Could you check a few things on this drawing? It's one solid part, dimensions in mm from its lowest x, y, z. A direction names the side the tool comes from. Round coordinates to 2 decimals unless told otherwise and drop trailing zeros. Write each loop counter-clockwise with the first axis right and the second up, starting at its lowest first coordinate (ties: lowest second). Pieces come first, ordered by that corner, then holes. Notation, with made-up numbers: M 75,2 L 86,2 A22 cw 86,18 Z; hole C 72.5,46 d5. An arc over 180 degrees is marked long. One line per item, written item: value. Start each with the question number.
(1) I want a section at D-D on y = 23. Please give me the cut outline in (x, z).
(2) If I drill on L1, parallel to X at y = 6, z = 135; L2, parallel to X at y = 1.45, z = 103; L3, parallel to Z at x = 10, y = 11.5, over which ranges is the centre line in solid material (lowest first)?
(3) I'm going to push flat-ended pins straight in: pin 1 Ø5 at (x, z) = (15.5, 42) entering from +Y; pin 2 Ø2.5 at (x, z) = (16, 103) entering from -Y; pin 3 Ø1 at (x, z) = (21.5, 145) entering from +Y. Where does each tip first touch, or does it pass through?
(4) I want a section at C-C on z = 103. Please give me the cut outline in (x, y).
(5) I want a section at B-B on y = 8. Please give me the cut outline in (x, z), and give its area (3 significant figures).
(6) Which directions (+Z, -Z, +X, -X, +Y, -Y) give clear straight access to the entire face, cutting with the end or side of a thin tool? Please do the marked faces 1 and 2.
(7) Thinking about a two-plate mould opening in X: for the marked faces 3, 4 and 5, which applies, released by +X, released by -X, zero draft, split by the parting line, or undercut?
(8) I want a section at A-A on x = 16. Please give me the cut outline in (y, z).
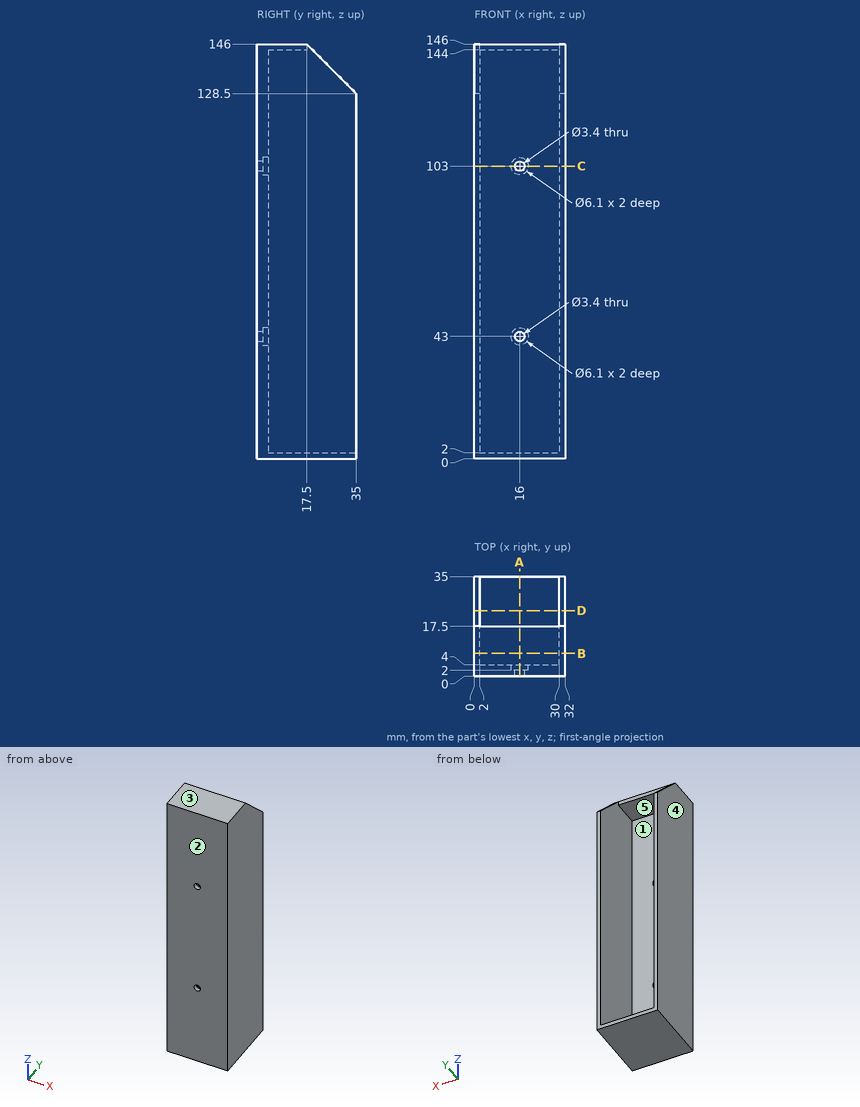
Found:
1. outline: M 0,0 L 32,0 L 32,140.5 L 30,140.5 L 30,2 L 2,2 L 2,140.5 L 0,140.5 Z
2. L1: x = 0 to 2, 30 to 32
2. L2: x = 0 to 14.3, 17.7 to 32
2. L3: z = 0 to 2, 144 to 146
3. pin 1: stops at y = 4
3. pin 2: passes through
3. pin 3: stops at y = 17.5
4. outline: M 0,0 L 14.3,0 L 14.3,2 L 12.95,2 L 12.95,4 L 2,4 L 2,35 L 0,35 Z; M 17.7,0 L 32,0 L 32,35 L 30,35 L 30,4 L 19.05,4 L 19.05,2 L 17.7,2 Z
5. outline: M 0,0 L 32,0 L 32,146 L 0,146 Z; hole M 2,2 L 30,2 L 30,144 L 2,144 Z
5. area: 696 mm²
6. face 1: +Y
6. face 2: +Z, -Z, +X, -X, -Y
7. face 3: zero draft
7. face 4: released by -X
7. face 5: undercut
8. outline: M 0,0 L 35,0 L 35,2 L 4,2 L 4,39.95 L 2,39.95 L 2,41.3 L 0,41.3 Z; M 0,44.7 L 2,44.7 L 2,46.05 L 4,46.05 L 4,99.95 L 2,99.95 L 2,101.3 L 0,101.3 Z; M 0,104.7 L 2,104.7 L 2,106.05 L 4,106.05 L 4,144 L 17.5,144 L 17.5,146 L 0,146 Z
